Build history of the part. All positions in model axes, mm. A direction names the side the tool comes from. Round coordinates to 2 decimals unless told otherwise and drop trailing zeros. Write each loop counter-clockwise with the first axis right and the second up, starting at its lowest first coordinate (ties: lowest second). Pieces come first, ordered by that corner, then holes.
1) Saw through at C-C (z = 10.5). Write the cut outline in (x, y), plus the area to 4 significant figures.
2) Saw through at A-A (y = 13). Write the cut outline in (x, z).
3) Wall check: probe 1 along Y at (x, z) = (-60, 23.75); probe 2 along Z at (x, y) = (-15.5, 42). Give the ranges that are in metal, low to high.
4) Saw through at D-D (x = 61.5). Write the cut outline in (y, z).
5) Which spindle directions (+Z, -Z, +X, -X, +Y, -Y) get a long thin tool onto all of the face, cutting with end or side? Do faces 1 (the flat face through (-34, 73, 25)), 2 (the cylindrical face through (53, -59, 1)), 3 (the flat face through (-1, -72.5, 14)). Say none if no direction does.
6) Pull direction X, two halves, no side cores. Call faces 4 (the flat face through (-1, 75, 12)), 5 (the cylindrical face through (54, 18, 1)), 6 (the flat face through (75, -1, 12)): +X half, -X half, draft (parallel to the pull), parting line (faces both ways), or undercut.
7) Saw through at B-B (x = 30). Write the cut outline in (y, z), plus the area to 4 significant figures.
from build123d import *

# Parameters (mm, degrees)
F0_W     = 150
F0_H     = 150
F1_DEPTH = 25
F2_T     = -2.5
F4_DEPTH = 25


with BuildPart() as f1:
    # F0 (on Top) → F1 (new body)
    with BuildSketch(Plane.XY):
        Rectangle(F0_W, F0_H)
    extrude(amount=F1_DEPTH)

    # F2
    f2_openings = [f1.faces().sort_by_distance(p)[0] for p in [
        (0, 0, 25),
    ]]
    offset(amount=F2_T, openings=f2_openings)

    # F3 (on face) → F4 (cut)
    with BuildSketch(Plane.XY.offset(2.5)):
        with BuildLine():
            Line((50, 20), (-50, 20))
            ThreePointArc((-50, 20), (-53.535534, 18.535534), (-55, 15))
            Line((-55, 15), (-55, -55))
            ThreePointArc((-55, -55), (-53.535534, -58.535534), (-50, -60))
            Line((-50, -60), (50, -60))
            ThreePointArc((50, -60), (53.535534, -58.535534), (55, -55))
            Line((55, -55), (55, 15))
            ThreePointArc((55, 15), (53.535534, 18.535534), (50, 20))
        make_face()
    extrude(amount=-F4_DEPTH, mode=Mode.SUBTRACT)


solid = f1.part
Evaluation:
1. outline: (-75, -75) - (75, -75) - (75, 75) - (-75, 75) - close; hole (-72.5, -72.5) - (72.5, -72.5) - (72.5, 72.5) - (-72.5, 72.5) - close
1. area: 1,475 mm2
2. outline: (-75, 0) - (-55, 0) - (-55, 2.5) - (-72.5, 2.5) - (-72.5, 25) - (-75, 25) - close; (55, 0) - (75, 0) - (75, 25) - (72.5, 25) - (72.5, 2.5) - (55, 2.5) - close
3. probe 1: y = -75 to -72.5, 72.5 to 75
3. probe 2: z = 0 to 2.5
4. outline: (-75, 0) - (75, 0) - (75, 25) - (72.5, 25) - (72.5, 2.5) - (-72.5, 2.5) - (-72.5, 25) - (-75, 25) - close
5. face 1: +Z, +X, -X, +Y, -Y
5. face 2: +Z, -Z
5. face 3: +Z
6. face 4: draft
6. face 5: undercut
6. face 6: +X half
7. outline: (-75, 0) - (-60, 0) - (-60, 2.5) - (-72.5, 2.5) - (-72.5, 25) - (-75, 25) - close; (20, 0) - (75, 0) - (75, 25) - (72.5, 25) - (72.5, 2.5) - (20, 2.5) - close
7. area: 287.5 mm2
